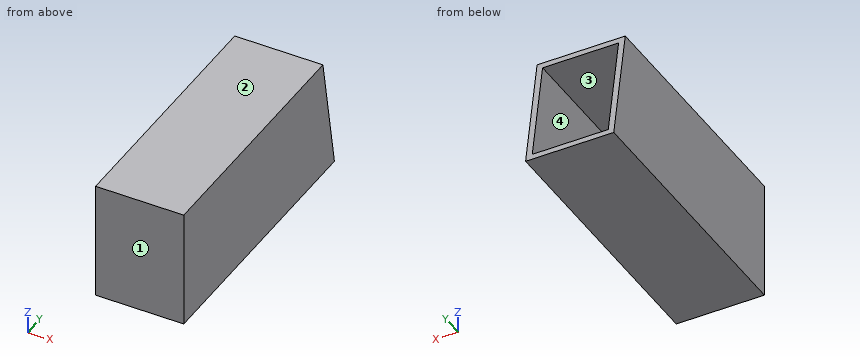
from build123d import *

# Parameters (mm, degrees)
SKETCH1_W               = 29
SKETCH1_H               = 39
BOSS_EXTRUDE1_DEPTH     = 90
SHELL1_T                = -2
CUT_EXTRUDE1_DEPTH      = 103.28391858
CUT_EXTRUDE1_DEPTH_BACK = 103.28391858


with BuildPart() as part:
    # Sketch1 → Boss-Extrude1 (new body)
    with BuildSketch(Plane(origin=(0, 0, 0), x_dir=(1, 0, 0), z_dir=(0, 1, 0))):
        with Locations((14.5, 19.5)):
            Rectangle(SKETCH1_W, SKETCH1_H)
    extrude(amount=BOSS_EXTRUDE1_DEPTH)

    # Shell1
    shell1_openings = [part.faces().sort_by_distance(p)[0] for p in [
        (14.5, 90, -19.5),
    ]]
    offset(amount=SHELL1_T, openings=shell1_openings, kind=Kind.INTERSECTION)

    # Sketch3 → Cut-Extrude1 (cut, two sides: drawn at the far end of the back side and taken through both)
    with BuildSketch(Plane.ZY.offset(-CUT_EXTRUDE1_DEPTH_BACK)):
        Polygon((-242.041155587, 125.801633924), (-39, 90), (0, 83.123247752), (203.041155587, 47.321613828), (274.644423436, 453.403925002), (-170.437887739, 531.883945099), align=None)
    extrude(amount=CUT_EXTRUDE1_DEPTH + CUT_EXTRUDE1_DEPTH_BACK, mode=Mode.SUBTRACT)


solid = part.part
The listing builds one solid part. Answer for the finished solid, in the listing's coordinates (mm). Face numbers are marked on the shaded views. Coordinates: 2 decimals unless noted, no trailing zeros. Loops run counter-clockwise (first coordinate to the right, second up) from the corner with the lowest first, then second, coordinate; pieces in that order, holes last.
1) Find section A-A on y = 36.5. Write down the section's boundary in (x, z).
2) Determine the mould class of the marked faces 1, 2, 3 and 4 for opening direction Z: pulls with the +Z half, pulls with the -Z half, needs draft (parallel to the pull), parting line crosses it, or undercut.
3) Find the intervals of material crossed by L1, parallel to X at y = 82.5, z = -21; L2, parallel to Z at x = 6.75, y = 31.5; L3, parallel to Y at x = 13.5, z = -17.5, in increasing order.
4) Find section B-B on x = 15.75. Write down the section's boundary in (y, z).
5) Find section C-C on z = -32. Write down the section's boundary in (x, y), then the cut area to 3 significant figures.
6) A flat-ended cylindrical pin translates along its axis: pin 1 Ø12.5 at (x, z) = (13, -22) entering from +Y. Find the tip coordinate at first contact, or state that the pin passes through.
Values:
1. outline: (0, -39) - (29, -39) - (29, 0) - (0, 0) - close; hole (2, -37) - (27, -37) - (27, -2) - (2, -2) - close
2. face 1: needs draft
2. face 2: pulls with the +Z half
2. face 3: undercut
2. face 4: undercut
3. L1: x = 0 to 2, 27 to 29
3. L2: z = -39 to -37, -2 to 0
3. L3: y = 0 to 2
4. outline: (0, -39) - (90, -39) - (89.65, -37) - (2, -37) - (2, -2) - (83.48, -2) - (83.12, 0) - (0, 0) - close
5. outline: (0, 0) - (29, 0) - (29, 88.77) - (27, 88.77) - (27, 2) - (2, 2) - (2, 88.77) - (0, 88.77) - close
5. area: 405 mm2
6. pin 1: stops at y = 2
